Input: part model. Units: mm. Frame: model coordinates. Face numbers are marked on the shaded views. Give positions to 0.01 mm unless a question says otherwise; leave off trailing zeros. Loops run counter-clockwise (first coordinate to the right, second up) from the corner with the lowest first, then second, coordinate; pieces in that order, holes last. Notation, with made-up numbers: M 17,45 L 51,45 A15 ccw 51,63 Z; hole C 69,-0.5 d4. An arc over 180 degrees is marked long. Return JSON: item names as keys, results as strings. Group by question number.
```python
from build123d import *

# Parameters (mm, degrees)
BOSS_EXTRUDE4_DEPTH       = 6
SKETCH1_10_R              = 3.7
SKETCH1_10_R_2            = 1.75
BOSS_EXTRUDE6_DEPTH       = 15
CUT_EXTRUDE1_START        = -6
CUT_EXTRUDE1_DEPTH        = 6
SKETCH6_R                 = 1.75
BOSS_EXTRUDE7_DEPTH       = 2
BOSS_EXTRUDE8_DEPTH       = 1
BOSS_EXTRUDE10_DEPTH      = 13
BOSS_EXTRUDE10_DEPTH_BACK = 6
CHAMFER2_SIZE             = 7
CUT_EXTRUDE2_DEPTH        = 1


with BuildPart() as part:
    # Sketch1 → Boss-Extrude4 (new body)
    with BuildSketch(Plane(origin=(0, 0, 0), x_dir=(1, 0, 0), z_dir=(0, 1, 0))):
        with BuildLine():
            Line((2.5, 4.330127019), (-14.820508076, 14.330127019))
            ThreePointArc((-14.820508076, 14.330127019), (-18.6051305, 14.794276156), (-21.650635095, 12.5))
            ThreePointArc((-21.650635095, 12.5), (-22.150137207, 8.705904774), (-19.820508076, 5.669872981))
            Line((-19.820508076, 5.669872981), (-2.5, -4.330127019))
            ThreePointArc((-2.5, -4.330127019), (4.330127019, -2.5), (2.5, 4.330127019))
        make_face()
    extrude(amount=BOSS_EXTRUDE4_DEPTH)

    # Sketch1<10> → Boss-Extrude6 (add)
    # profile 1 of 2: a face of its own
    with BuildSketch(Plane(origin=(0, 0, 0), x_dir=(1, 0, 0), z_dir=(0, 1, 0))):
        with Locations(Location((0, 0, 0), (0, 0, 270))):
            Circle(SKETCH1_10_R)
        with Locations(Location((0, 0, 0), (0, 0, 270))):
            Circle(SKETCH1_10_R_2, mode=Mode.SUBTRACT)
    # profile 2 of 2: a face of its own
    with BuildSketch(Plane(origin=(0, 0, 0), x_dir=(1, 0, 0), z_dir=(0, 1, 0))):
        with Locations(Location((-17.320508076, 10, 0), (0, 0, 270))):
            Circle(SKETCH1_10_R)
        with Locations(Location((-17.320508076, 10, 0), (0, 0, 270))):
            Circle(SKETCH1_10_R_2, mode=Mode.SUBTRACT)
    extrude(amount=BOSS_EXTRUDE6_DEPTH)

    # Sketch5 → Cut-Extrude1 (cut)
    with BuildSketch(Plane(origin=(0, 15, 0), x_dir=(1, 0, 0), z_dir=(0, 1, 0)).offset(CUT_EXTRUDE1_START)):
        with BuildLine():
            Line((-20.014101509, 12.536642351), (-18.220272206, 11.50097452))
            ThreePointArc((-18.220272206, 11.50097452), (-18.836052532, 10.875), (-19.070272206, 10.028731334))
            Line((-19.070272206, 10.028731334), (-20.864101509, 11.064399165))
            ThreePointArc((-20.864101509, 11.064399165), (-20.52480207, 11.85), (-20.014101509, 12.536642351))
        make_face()
        with BuildLine():
            Line((-13.776914643, 8.935600835), (-15.570743946, 9.971268666))
            ThreePointArc((-15.570743946, 9.971268666), (-15.804963619, 9.125), (-16.420743946, 8.49902548))
            Line((-16.420743946, 8.49902548), (-14.626914643, 7.463357649))
            ThreePointArc((-14.626914643, 7.463357649), (-14.116214082, 8.15), (-13.776914643, 8.935600835))
        make_face()
        with BuildLine():
            Line((2.693593433, -2.536642351), (0.89976413, -1.50097452))
            ThreePointArc((0.89976413, -1.50097452), (1.515544457, -0.875), (1.74976413, -0.028731334))
            Line((1.74976413, -0.028731334), (3.543593433, -1.064399165))
            ThreePointArc((3.543593433, -1.064399165), (3.204293994, -1.85), (2.693593433, -2.536642351))
        make_face()
        with BuildLine():
            Line((-3.543593433, 1.064399165), (-1.74976413, 0.028731334))
            ThreePointArc((-1.74976413, 0.028731334), (-1.515544457, 0.875), (-0.89976413, 1.50097452))
            Line((-0.89976413, 1.50097452), (-2.693593433, 2.536642351))
            ThreePointArc((-2.693593433, 2.536642351), (-3.204293994, 1.85), (-3.543593433, 1.064399165))
        make_face()
    extrude(amount=CUT_EXTRUDE1_DEPTH, mode=Mode.SUBTRACT)

    # Sketch6 → Boss-Extrude7 (add)
    with BuildSketch(Plane(origin=(0, 6, 0), x_dir=(1, 0, 0), z_dir=(0, 1, 0))):
        with Locations(Location((-17.320508076, 10, 0), (0, 0, 120.940718932))):
            Circle(SKETCH6_R)
        with Locations(Location((0, 0, 0), (0, 0, 90))):
            Circle(SKETCH6_R)
    extrude(amount=BOSS_EXTRUDE7_DEPTH)

    # Sketch8 → Boss-Extrude8 (add)
    with BuildSketch(Plane(origin=(0, 15, 0), x_dir=(1, 0, 0), z_dir=(0, 1, 0))):
        with BuildLine():
            Line((-18.220272206, 11.50097452), (-20.447114211, 12.786642351))
            ThreePointArc((-20.447114211, 12.786642351), (-15.161166743, 13.7400889), (-13.343901941, 8.685600835))
            Line((-13.343901941, 8.685600835), (-15.570743946, 9.971268666))
            ThreePointArc((-15.570743946, 9.971268666), (-16.445508076, 11.515544457), (-18.220272206, 11.50097452))
        make_face()
        with BuildLine():
            Line((-16.420743946, 8.49902548), (-14.193901941, 7.213357649))
            ThreePointArc((-14.193901941, 7.213357649), (-19.479849409, 6.2599111), (-21.297114211, 11.314399165))
            Line((-21.297114211, 11.314399165), (-19.070272206, 10.028731334))
            ThreePointArc((-19.070272206, 10.028731334), (-18.195508076, 8.484455543), (-16.420743946, 8.49902548))
        make_face()
        with BuildLine():
            Line((0.89976413, -1.50097452), (3.126606135, -2.786642351))
            ThreePointArc((3.126606135, -2.786642351), (-2.159341333, -3.7400889), (-3.976606135, 1.314399165))
            Line((-3.976606135, 1.314399165), (-1.74976413, 0.028731334))
            ThreePointArc((-1.74976413, 0.028731334), (-0.875, -1.515544457), (0.89976413, -1.50097452))
        make_face()
        with BuildLine():
            Line((-0.89976413, 1.50097452), (-3.126606135, 2.786642351))
            ThreePointArc((-3.126606135, 2.786642351), (2.159341333, 3.7400889), (3.976606135, -1.314399165))
            Line((3.976606135, -1.314399165), (1.74976413, -0.028731334))
            ThreePointArc((1.74976413, -0.028731334), (0.875, 1.515544457), (-0.89976413, 1.50097452))
        make_face()
    extrude(amount=BOSS_EXTRUDE8_DEPTH)

    # Sketch1<12> → Boss-Extrude10 (add, two sides: drawn at the far end of the back side and taken through both)
    with BuildSketch(Plane(origin=(0, 0, 0), x_dir=(1, 0, 0), z_dir=(0, 1, 0)).offset(-BOSS_EXTRUDE10_DEPTH_BACK)):
        with BuildLine():
            Line((-34.490381057, 29.739092363), (-37.990381057, 35.801270189))
            ThreePointArc((-37.990381057, 35.801270189), (-23.350583329, 28.362250924), (-14.820508076, 14.330127019))
            ThreePointArc((-14.820508076, 14.330127019), (-18.6051305, 14.794276156), (-21.650635095, 12.5))
            ThreePointArc((-21.650635095, 12.5), (-26.123146339, 22.569949107), (-34.490381057, 29.739092363))
        make_face()
    extrude(amount=BOSS_EXTRUDE10_DEPTH + BOSS_EXTRUDE10_DEPTH_BACK)

    # Chamfer2
    # the kernel refuses this chamfer: 7 mm, written as the material it takes off along each edge
    with BuildSketch(Plane(origin=(-17.287458299, -6, -9.876656552), x_dir=(0.2618523083710211, 0, 0.9651079569668709), z_dir=(-0.9651079569668709, 0, 0.2618523083710211))) as chamfer2_piece_1_section:
        Polygon((5.09109444 + CHAMFER2_SIZE, 0), (5.09109444, CHAMFER2_SIZE), (5.09109444, 0), align=None)
    chamfer2_piece_1 = revolve(axis=Axis((-17.287458299, -6, -9.876656552), (0, 1, 0)), revolution_arc=359.64, mode=Mode.PRIVATE)
    chamfer2_piece_1 = split(chamfer2_piece_1, bisect_by=Plane(origin=(-19.646446417, 0, -18.680520064), z_dir=(0, -1, 0)), keep=Keep.TOP, mode=Mode.PRIVATE)
    add(chamfer2_piece_1, mode=Mode.SUBTRACT)
    with BuildSketch(Plane(origin=(-17.287458299, 13, -9.876656552), x_dir=(0.2618523083710211, 0, 0.9651079569668709), z_dir=(-0.9651079569668709, 0, 0.2618523083710211))) as chamfer2_piece_2_section:
        Polygon((5.09109444 + CHAMFER2_SIZE, 0), (5.09109444, -CHAMFER2_SIZE), (5.09109444, 0), align=None)
    chamfer2_piece_2 = revolve(axis=Axis((-17.287458299, 13, -9.876656552), (0, 1, 0)), revolution_arc=359.64, mode=Mode.PRIVATE)
    chamfer2_piece_2 = split(chamfer2_piece_2, bisect_by=Plane(origin=(-19.516900024, 6, -18.197046345), z_dir=(0, 1, 0)), keep=Keep.TOP, mode=Mode.PRIVATE)
    add(chamfer2_piece_2, mode=Mode.SUBTRACT)

    # Sketch9 → Cut-Extrude2 (cut)
    with BuildSketch(Plane(origin=(0, 16, 0), x_dir=(1, 0, 0), z_dir=(0, 1, 0))):
        Polygon((-20.864101509, 11.064399165), (-21.559190629, 9.860469492), (-22.101511133, 10.173578381), (-21.406422012, 11.377508053), align=None)
        Polygon((-20.014101509, 12.536642351), (-19.319012388, 13.740572024), (-19.910294762, 14.081949062), (-20.605383883, 12.878019389), align=None)
        Polygon((-12.490543148, 9.79815347), (-13.081825522, 10.139530508), (-13.776914643, 8.935600835), (-13.185632268, 8.594223797), align=None)
        Polygon((-14.084594139, 7.15024876), (-14.626914643, 7.463357649), (-15.322003763, 6.259427976), (-14.77968326, 5.946319087), align=None)
        Polygon((-3.543593433, 1.064399165), (-4.238682554, -0.139530508), (-4.781003057, 0.173578381), (-4.085913936, 1.377508053), align=None)
        Polygon((-2.693593433, 2.536642351), (-1.998504312, 3.740572024), (-2.589786687, 4.081949062), (-3.284875807, 2.878019389), align=None)
        Polygon((4.829964928, -0.20184653), (4.238682554, 0.139530508), (3.543593433, -1.064399165), (4.134875807, -1.405776203), align=None)
        Polygon((3.235913936, -2.84975124), (2.693593433, -2.536642351), (1.998504312, -3.740572024), (2.540824816, -4.053680913), align=None)
    extrude(amount=-CUT_EXTRUDE2_DEPTH, mode=Mode.SUBTRACT)


solid = part.part
```
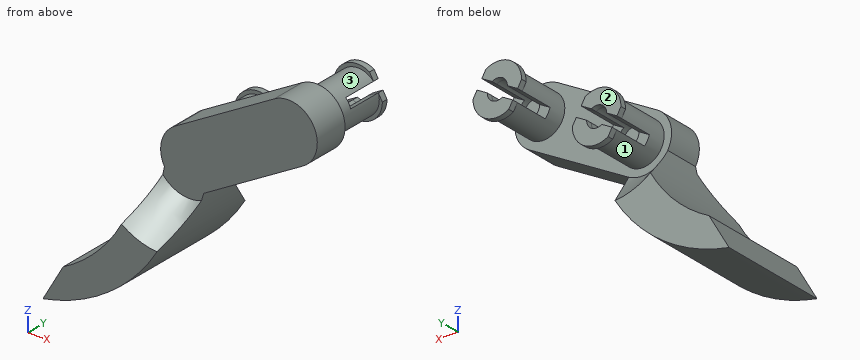
Item 1: Section D-D, the plane x = -33.5. Return loops of the section in (y, z).
Item 2: Material intervals for line 1 (X direction, y = 11.5, z = 0); line 2 (Y direction, x = -18.5, z = -11), sorted ascending. Write a range as from..to.
Item 3: Section A-A, the plane y = 5. Return loops of the section in (x, z), then the cut area to 3 significant figures.
Item 4: First-contact query: pin 1 Ø4.5 at (x, z) = (0, 0) entering from -Y; pin 2 Ø3 at (y, z) = (9.5, -11.5) entering from +X; pin 3 Ø2 at (x, y) = (-33, -3.5) entering from +Z. Flat tips, straight axial feed; report the tip coordinate or a pass-through.
Item 5: Section B-B, the plane x = 0. Return loops of the section in (y, z), then the cut area to 3 significant figures.
Item 6: Pull-direction query (Z, two-part tool) for the marked faces 1, 2 and 3; classes: pulls with the +Z half, pulls with the -Z half, needs draft (parallel to the pull), parting line crosses it, or undercut.
Item 7: Section C-C, the plane z = -23.5. Return loops of the section in (x, y).
Answer below:
{
 "1": {"outline": "M -6,-34.56 L 13,-34.56 L 13,-29.19 L -6,-29.19 Z"},
 "2": {"line 1": "-3.7..-1.75, 1.75..3.7", "line 2": "0..8"},
 "3": {"outline": "M -37.99,-35.8 A30 ccw -14.82,-14.33 L 2.5,-4.33 A5 ccw -2.5,4.33 L -19.82,-5.67 A5 ccw -21.65,-12.5 A25 cw -34.49,-29.74 Z", "area": "436 mm^2"},
 "4": {"pin 1": "y = 0", "pin 2": "x = -13.62", "pin 3": "z = -28.23"},
 "5": {"outline": "M 0,-5.77 L 6,-5.77 L 6,-3.7 L 15,-3.7 L 15,-4.3 L 16,-4.3 L 16,-1.75 L 8,-1.75 L 8,1.75 L 16,1.75 L 16,4.3 L 15,4.3 L 15,3.7 L 6,3.7 L 6,5 L 0,5 Z", "area": "112 mm^2"},
 "6": {"face 1": "undercut", "face 2": "needs draft", "face 3": "parting line crosses it"},
 "7": {"outline": "M -26.85,-6 L -19.12,-6 L -19.12,13 L -26.85,13 Z"}
}
